from build123d import *

# Parameters (mm, degrees)
BOSS_EXTRUDE1_DEPTH = 3
BOSS_EXTRUDE3_DEPTH = 3
BOSS_EXTRUDE4_START = -10
BOSS_EXTRUDE4_DEPTH = 410


with BuildPart() as part:
    # 3DSketch1 → Boss-Extrude1 (new body)
    with BuildSketch(Plane(origin=(-317.933582459, 130.294447415, 321.791546701), x_dir=(0.6513102781690263, 0, 0.7588115191214388), z_dir=(0, -1, 0))):
        Polygon((0, 0), (353.62249966, 303.524607649), (614.146610928, 0), (260.524111268, -303.524607649), align=None)
    extrude(amount=-BOSS_EXTRUDE1_DEPTH)



with BuildPart() as body_2:
    # Sketch2 → Boss-Extrude3 (new body)
    with BuildSketch(Plane(origin=(0, 441.171604384, 528.116012859), x_dir=(1, 0, 0), z_dir=(0, 0.6411058174679163, 0.7674524941706782))):
        Polygon((-317.933582459, -614.057029458), (-317.933582459, -405.07674329), (82.066417541, -405.07674329), (82.066417541, -504.870685967), (32.066417541, -504.870685967), (32.066417541, -614.057029458), align=None)
    extrude(amount=BOSS_EXTRUDE3_DEPTH)


with BuildPart() as part_1:
    add(part.part)

    add(body_2.part)  # Boss-Extrude4 merges body 2
    # Sketch3 → Boss-Extrude4 (add)
    with BuildSketch(Plane.ZY.offset(327.933582459).offset(BOSS_EXTRUDE4_START)):
        Polygon((787.813069503, 130.294447415), (787.813069503, 133.294447415), (790.115426985, 132.217764868), align=None)
    extrude(amount=-BOSS_EXTRUDE4_DEPTH)


solid = part_1.part
Could you check a few things on this model? Use its own coordinates, in mm. A direction names the side the tool comes from. Give positions to 0.01 mm unless a question says otherwise; leave off trailing zeros. Order: outer loops, then holes, each group sorted by start corner. A loop starts at its lowest first (then second) coordinate and runs counter-clockwise, first axis right, second up.
1. Suppose I cut it at B-B (z = 643). Write out the boundary of the cut face in (x, y).
Answers below:
outline: (-317.93, 130.29) - (82.07, 130.29) - (82.07, 133.29) - (-317.93, 133.29) - close
2. For pin 1 (1 mm diameter, centred on x = -132, y = 41, fed in from -Z); pin 2 (12 mm diameter, centred on x = -211.5, z = 615, fed in from -Y); pin 3 (1.5 mm diameter, centred on x = 85, y = 131.5, fed in from -Z), each with a flat end and sliding along its axis, tell me the tip position at first contact or that it passes through.
Answers below:
pin 1: stops at z = 861.99
pin 2: stops at y = 130.29
pin 3: stops at z = 787.81
3. Suppose I cut it at D-D (y = 24.5). Write out the boundary of the cut face in (x, z).
Answers below:
outline: (-317.93, 876.19) - (32.07, 876.19) - (32.07, 880.1) - (-317.93, 880.1) - close
4. I need wall thicknesses on L1, parallel to Y at x = 2.5, z = 358.5; L2, parallel to Z at x = -261.5, y = 116; L3, parallel to Z at x = 1, y = 85. Which ranges of each line are inside material? Lowest first, please.
Answers below:
L1: y = 130.29 to 133.29
L2: z = 799.75 to 803.66
L3: z = 825.65 to 829.56
5. Which directions (+Z, -Z, +X, -X, +Y, -Y) give clear straight access to the entire face, cutting with the end or side of a thin tool? Please do faces 1 (the flat face through (-115.134, 53.149, 856.167)), 2 (the flat face through (-118, 130.294, 561)).
Answers below:
face 1: +Z, +X, -X, +Y
face 2: -Z, +X, -X, -Y
6. Suppose I cut it at C-C (x = -183.5). Write out the boundary of the cut face in (y, z).
Answers below:
outline: (-30.09, 921.79) - (130.29, 787.81) - (130.29, 321.79) - (133.29, 321.79) - (133.29, 787.81) - (132.22, 790.12) - (-28.16, 924.09) - close
7. Suppose I cut it at A-A (x = 61). Write out the boundary of the cut face in (y, z).
Answers below:
outline: (53.71, 851.79) - (130.29, 787.81) - (130.29, 321.79) - (133.29, 321.79) - (133.29, 787.81) - (132.22, 790.12) - (55.63, 854.09) - close
